For this review, take the finished solid that the model builds, in its own axes (mm). Face numbers are marked on the shaded views. Coordinates: 2 decimals unless noted, no trailing zeros. Write each loop counter-clockwise with the first axis right and the second up, starting at its lowest first coordinate (ties: lowest second). Pieces come first, ordered by that corner, then holes. Notation, with made-up numbers: (-25, -20.75) -> (13, -20.75) arc R11 ccw to (13, -1.75) -> close; hole circle Ø10 at (68, 24). An arc over 180 degrees is marked (long way). One line per item, written item: value. Start each with the question number.
1) For probe 1 along X at (y, z) = (-0.5, -14); probe 2 along X at (y, z) = (-16, -8), list the stretches that pass through material, from the lowest coordinate up. Write a range as from..to.
2) Add section A-A (y = 0). State the section outline as (x, z) points (3 decimals).
3) Mouldability with a two-part tool opening along Y and no side actions: class the marked faces 1, 2 and 3 as released by +Y, released by -Y, zero draft, split by the parting line, or undercut.
4) For pin 1 Ø1.6 at (x, z) = (49, -4) entering from +Y; pin 2 Ø4 at (x, y) = (-10, 2) entering from +Z; pin 3 Ø1.9 at (x, y) = (47.5, 0.5) entering from +Z; pin 4 Ø0.6 at (x, z) = (34.5, -0.5) entering from -Y, all flat-tipped, find the tip position at first contact; note any pin that passes through.
Autodesk Inventor part; units mm, degrees
ref_plane "YZ Plane" through (0, 0, 0) normal (1, 0, 0) x (0, 1, 0)
ref_plane "XZ Plane" through (0, 0, 0) normal (0, 1, 0) x (-1, 0, 0)
ref_plane "XY Plane" through (0, 0, 0) normal (0, 0, 1) x (1, 0, 0)
sketch "FishmanModern8" plane through (0, 0, 0) normal (0, 0, 1) x (1, 0, 0)
  line L0 (-50.9143, 0) -> (50.9143, 0) construction
  line L1 (0, 18.9484) -> (0, -18.9484) construction
  line L2 (-50.9143, 18.9484) -> (50.9143, 18.9484)
  line L3 (50.9143, 18.9484) -> (50.9143, -18.9484)
  line L4 (50.9143, -18.9484) -> (-50.9143, -18.9484)
  line L5 (-50.9143, -18.9484) -> (-50.9143, 18.9484)
  circle A0 centre (-47.625, 0) radius 1.27
  circle A1 centre (47.625, 0) radius 1.27
  line L6 (-3.3542, -4.7903) -> (3.3542, 4.7903)
  line L7 (-6.3503, -6.35) -> (-50.9143, -6.35)
  line L8 (6.3503, 6.35) -> (50.9143, 6.35)
  circle A2 centre (-47.625, 0) radius 3.175
  circle A3 centre (47.625, 0) radius 3.175
  line L9 (-50.9143, 3.175) -> (-47.625, 3.175)
  line L10 (-50.9143, -3.175) -> (-47.625, -3.175)
  line L11 (47.625, 3.175) -> (50.9143, 3.175)
  line L12 (47.625, -3.175) -> (50.9143, -3.175)
  arc A4 (6.3503, 6.35) -> (3.3542, 4.7903) centre (6.3503, 2.6924) ccw
  arc A5 (-6.3503, -6.35) -> (-3.3542, -4.7903) centre (-6.3503, -2.6924) ccw
  line L13 (50.9143, 6.731) -> (6.3503, 6.731)
  arc A6 (6.3503, 6.731) -> (3.0421, 5.0088) centre (6.3503, 2.6924) ccw
  line L14 (3.0421, 5.0088) -> (-3.6663, -4.5718)
  arc A7 (-6.3503, -5.969) -> (-3.6663, -4.5718) centre (-6.3503, -2.6924) ccw
  line L15 (-6.3503, -5.969) -> (-50.9143, -5.969)
  line L16 (50.9143, 5.969) -> (6.3503, 5.969)
  arc A8 (6.3503, 5.969) -> (3.6663, 4.5718) centre (6.3503, 2.6924) ccw
  line L17 (3.6663, 4.5718) -> (-3.0421, -5.0088)
  arc A9 (-6.3503, -6.731) -> (-3.0421, -5.0088) centre (-6.3503, -2.6924) ccw
  line L18 (-6.3503, -6.731) -> (-50.9143, -6.731)
  line L19 (-50.9143, -5.969) -> (-50.9143, -6.731)
  line L20 (50.9143, 6.731) -> (50.9143, 5.969)
  point P0 (0, 0)
  point P1 (0, 0)
  dimension "d72" = 101.8286
  dimension "d73" = 37.8968
  dimension "d74" = 2.54
  dimension "d75" = 95.25
  dimension "d76" = 47.625
  dimension "d77" = 47.625
  dimension "d78" = 55
  dimension "d79" = 6.35
  dimension "d80" = 6.35
  dimension "d81" = 6.35
  dimension "d85" = 3.6576
  dimension "d86" = 0.381
  dimension "d87" = 0.381
extrude "FishmanModern8Feature" add sketch "FishmanModern8" against normal blind 18.0086 contours L2 L3 L13 A6 L14 A7 L15 L5 L10 A2 L9 | L9 A2 L10 L5 | L3 L8 A4 L6 A5 L7 L5 L15 A7 L14 A6 L13 | A2 | L3 L16 A8 L17 A9 L18 L5 L7 A5 L6 A4 L8 | L3 L11 A3 L12 L4 L5 L18 A9 L17 A8 L16 | L3 L12 A3 L11 | A3 | A0 | A1
fillet "FishmanModern8FilletsFeature" radius 3.6576 4 edges at (-50.9143, 18.9484, -9.0043) (-50.9143, -18.9484, -9.0043) (50.9143, 18.9484, -9.0043) (50.9143, -18.9484, -9.0043)
extrude "FishmanModern8IndentFeature" cut sketch "FishmanModern8" against normal blind 1.27 contours L3 L8 A4 L6 A5 L7 L5 L15 A7 L14 A6 L13 | L3 L16 A8 L17 A9 L18 L5 L7 A5 L6 A4 L8
extrude "FishmanModern8MountsFeature" cut sketch "FishmanModern8" against normal through all contours A0 | A1
extrude "FishmanModern8CountersinksFeature" cut sketch "FishmanModern8" against normal blind 6.35 contours L9 A2 L10 L5 | A2 | L3 L12 A3 L11 | A3 | A1
chamfer "FishmanModern8ChamferFeature" distance 1.27 angle 45 12 edges at (0, 18.9484, 0) (-49.843, 17.8771, 0) (-50.9143, 9.2329, 0) (49.843, 17.8771, 0) (50.9143, 11.0109, 0) (0, -18.9484, 0) (49.843, -17.8771, 0) (50.9143, -9.2329, 0) (-49.843, -17.8771, 0) (-50.9143, -11.0109, 0) (-50.9143, -4.572, 0) (50.9143, 4.572, 0)
equation "\"d76\" = d77"
properties part number "fishman-modern8"
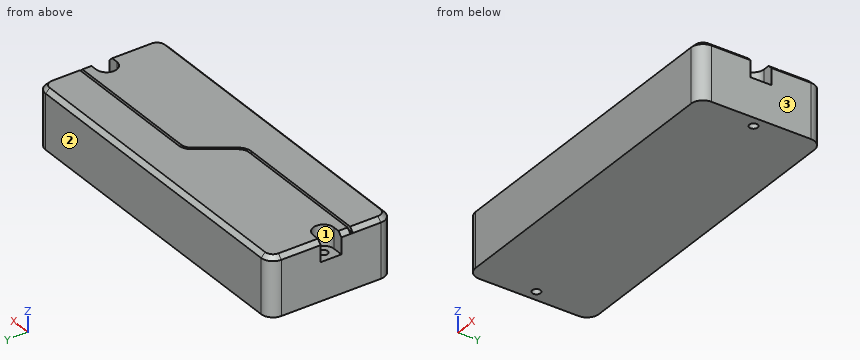
Numbers:
1. probe 1: -50.91..-48.79, -46.46..46.46, 48.79..50.91
1. probe 2: -50.84..50.84
2. outline: (-50.914, -18.009) -> (-48.895, -18.009) -> (-48.895, -6.35) -> (-50.914, -6.35) -> close; (-46.355, -18.009) -> (46.355, -18.009) -> (46.355, -6.35) -> (44.45, -6.35) -> (44.45, 0) -> (0.465, 0) -> (0.465, -1.27) -> (-0.465, -1.27) -> (-0.465, 0) -> (-44.45, 0) -> (-44.45, -6.35) -> (-46.355, -6.35) -> close; (48.895, -18.009) -> (50.914, -18.009) -> (50.914, -6.35) -> (48.895, -6.35) -> close
3. face 1: undercut
3. face 2: released by +Y
3. face 3: zero draft
4. pin 1: y = 18.82
4. pin 2: z = 0
4. pin 3: z = -6.35
4. pin 4: y = -18.48
